Geometry: final body of the model. Coordinates: model frame, mm. A direction names the side the tool comes from. Round coordinates to 2 decimals unless told otherwise and drop trailing zeros. Write each loop counter-clockwise with the first axis right and the second up, starting at its lowest first coordinate (ties: lowest second). Pieces come first, ordered by that corner, then holes. Notation, with made-up numbers: M -6.5,-19 L 42.5,-19 A19 ccw 42.5,-6 Z; hole C -36,27.25 d5. An arc over 180 degrees is marked long. Use one line per item in the form item = value. Start each with the question number.
Item 1: Section query D-D (x = -19.25). Return loops of the section in (y, z).
Item 2: Ray query, probe 1 along Z at (x, y) = (-0.6, -28.5); probe 2 along X at (y, z) = (25.5, 4); probe 3 along Z at (x, y) = (-4.5, 11.5). Return the intervals inside material, ascending.
Item 3: Pin query (flat end, axial travel): pin 1 Ø1.5 at (x, z) = (-19.5, 3.5) entering from +Y; pin 2 Ø5.5 at (x, y) = (-9.5, -8.5) entering from +Z; pin 3 Ø5 at (x, z) = (-16, 7.5) entering from +Y. Return the tip coordinate at first contact, or that it passes through.
Item 4: Reachability of faces 4 (the cylindrical face through (-17.096, -0.375, 2.493)), 5 (the cylindrical face through (-18.096, 0.397, 2.493)), 6 (the flat face through (-2, 28, 7)), 7 (the flat face through (-2, -28, 7)) from +Z, -Z, +X, -X, +Y, -Y: full face, straight path, thin tool, end or side. Return the list, or none.
Item 5: Section query C-C (y = 28.5). Return loops of the section in (x, z), and give its area (3 significant figures).
Item 6: Pull-direction query (Z, two-part tool) for faces 1 (the flat face through (-17, -3, 3)), 2 (the flat face through (-0.1, -24, 4)), 3 (the cylindrical face through (-1.04, -29.77, 4.03)); classes: pulls with the +Z half, pulls with the -Z half, needs draft (parallel to the pull), parting line crosses it, or undercut.
from build123d import *

# Parameters (mm, degrees)
BOSS_EXTRUDE1_DEPTH = 2
BOSS_EXTRUDE2_DEPTH = 10
BOSS_EXTRUDE3_DEPTH = 10
SKETCH3_R           = 1.6
CUT_EXTRUDE1_DEPTH  = 10
BOSS_EXTRUDE4_DEPTH = 1
MOVE_FACE1_DEPTH    = 10
BOSS_EXTRUDE5_DEPTH = 1


# Read off the part's stored shape, not the designer's step: Move Face1
with BuildPart() as part:
    # Sketch1 → Boss-Extrude1 (new body)
    with BuildSketch(Plane.XY):
        with BuildLine():
            Line((0, 23), (0, 2.65))
            ThreePointArc((0, 2.65), (-2.65, 0), (0, -2.65))
            Line((0, -2.65), (0, -23))
            ThreePointArc((0, -23), (-23, 0), (0, 23))
        make_face()
    extrude(amount=BOSS_EXTRUDE1_DEPTH)

    # Sketch2 → Boss-Extrude2 (add)
    with BuildSketch(Plane.XY):
        with BuildLine():
            Line((0, 23), (0, 24.5))
            ThreePointArc((0, 24.5), (-24.5, 0), (0, -24.5))
            Line((0, -24.5), (0, -23))
            ThreePointArc((0, -23), (-23, 0), (0, 23))
        make_face()
    extrude(amount=BOSS_EXTRUDE2_DEPTH)

    # Sketch4 → Boss-Extrude3 (add)
    with BuildSketch(Plane.XY.offset(10)):
        Polygon((0, -24.5), (-0.271688165, -23.208442848), (-2, -23.208442848), (-2, -32.5), (0, -32.5), align=None)
    boss_extrude3 = extrude(amount=-BOSS_EXTRUDE3_DEPTH)

    # Sketch3 → Cut-Extrude1 (cut)
    with BuildSketch(Plane(origin=(0, 0, 0), x_dir=(0, 0, -1), z_dir=(1, 0, 0))):
        with Locations(Location((-5, -28.5, 0), (0, 0, 90))):
            Circle(SKETCH3_R)
    cut_extrude1 = extrude(amount=-CUT_EXTRUDE1_DEPTH, mode=Mode.SUBTRACT)

    # Sketch5 → Boss-Extrude4 (add)
    with BuildSketch(Plane(origin=(0, 0, 0), x_dir=(-1, 0, 0), z_dir=(0, 0, -1))):
        Polygon((2, -32.5), (9.124047282, -22.73767273), (2, -22.73767273), align=None)
    boss_extrude4 = extrude(amount=-BOSS_EXTRUDE4_DEPTH)

    # Mirror1: Boss-Extrude3, Cut-Extrude1, Boss-Extrude4 across plane
    add(boss_extrude3.mirror(Plane.ZX))
    add(cut_extrude1.mirror(Plane.ZX), mode=Mode.SUBTRACT)
    add(boss_extrude4.mirror(Plane.ZX))

    # Move Face1 outline → Move Face1 (cut)
    with BuildSketch(Plane.XY):
        with BuildLine():
            ThreePointArc((-0.1, 2.748181217), (-2.75, 0), (-0.1, -2.748181217))
            Line((-0.1, -2.748181217), (-0.1, -32.5))
            Line((-0.1, -32.5), (0, -32.5))
            Line((0, -32.5), (0, -2.65))
            ThreePointArc((0, -2.65), (-2.65, 0), (0, 2.65))
            Line((0, 2.65), (0, 32.5))
            Line((0, 32.5), (-0.1, 32.5))
            Line((-0.1, 32.5), (-0.1, 2.748181217))
        make_face()
    extrude(amount=MOVE_FACE1_DEPTH, mode=Mode.SUBTRACT)

    # Sketch6 → Boss-Extrude5 (add)
    with BuildSketch(Plane.XY.offset(2)):
        with BuildLine():
            Line((-0.1, 17.0997076), (-0.1, 18.099723755))
            ThreePointArc((-0.1, 18.099723755), (-18.1, 0), (-0.1, -18.099723755))
            Line((-0.1, -18.099723755), (-0.1, -17.0997076))
            ThreePointArc((-0.1, -17.0997076), (-17.1, 0), (-0.1, 17.0997076))
        make_face()
    extrude(amount=BOSS_EXTRUDE5_DEPTH)


solid = part.part
Working result:
q1.outline = M -15.16,0 L 15.16,0 L 15.16,10 L 12.59,10 L 12.59,2 L -12.59,2 L -12.59,10 L -15.16,10 Z
q2.probe_1 = 0 to 3.4, 6.6 to 10
q2.probe_2 = -2 to -0.1
q2.probe_3 = 0 to 2
q3.pin_1 = 15.77
q3.pin_2 = 2
q3.pin_3 = 20.45
q4.face_4 = +Z, +X
q4.face_5 = +Z
q4.face_6 = +Z, -X, +Y
q4.face_7 = +Z, -X, -Y
q5.outline = M -4.92,0 L -0.1,0 L -0.1,3.4 L -2,3.4 L -2,1 L -4.92,1 Z; M -2,6.6 L -0.1,6.6 L -0.1,10 L -2,10 Z
q5.area = 15.8 mm²
q6.face_1 = pulls with the +Z half
q6.face_2 = needs draft
q6.face_3 = undercut
